from build123d import *

# Parameters (mm, degrees)
SKICA1_W                = 7.9
SKICA1_H                = 3
P_IDAT_VYSUNUT_M1_DEPTH = 2.3
SKICA2_R                = 1
P_IDAT_VYSUNUT_M2_DEPTH = 2.5
ZKOSEN_2_SIZE           = 0.7


with BuildPart() as part:
    # Skica1 → Přidat vysunutím1 (new body)
    with BuildSketch(Plane.XY):
        Rectangle(SKICA1_W, SKICA1_H)
    extrude(amount=P_IDAT_VYSUNUT_M1_DEPTH)

    # Skica2 → Přidat vysunutím2 (add)
    with BuildSketch(Plane.XY.offset(2.3)):
        with Locations((-2.3, 0)):
            Circle(SKICA2_R)
        with Locations((2.3, 0)):
            Circle(SKICA2_R)
    extrude(amount=P_IDAT_VYSUNUT_M2_DEPTH)

    # Zkosení2
    zkosen_2_edges = [part.edges().sort_by_distance(p)[0] for p in [
        (-3.3, 0, 4.8),
        (1.3, 0, 4.8),
    ]]
    chamfer(zkosen_2_edges, length=ZKOSEN_2_SIZE)


solid = part.part
Input: part model. Units: mm. Frame: model coordinates. A direction names the side the tool comes from. Coordinates: 2 decimals unless noted, no trailing zeros. Loops run counter-clockwise (first coordinate to the right, second up) from the corner with the lowest first, then second, coordinate; pieces in that order, holes last. Notation, with made-up numbers: (-20.75, -2.5) -> (-6.75, -2.5) arc R16 cw to (-6.75, 20.5) -> close; hole circle Ø8 at (11.5, 45.5). An arc over 180 degrees is marked (long way). Write each question's results on one line, items separated by ' | '. Start each with the question number.
Q1. Pin query (flat end, axial travel): pin 1 (0.9 mm diameter, centred on x = 0.5, y = 0, fed in from +Z). Return the tip coordinate at first contact, or that it passes through.
Q2. Reachability of faces 1 (the cylindrical face through (-3.3, 0, 3.2)), 2 (the flat face through (3.95, 0, 1)) from +Z, -Z, +X, -X, +Y, -Y: full face, straight path, thin tool, end or side. Return the list, or none.
Q3. Section A-A, the plane y = 0. Return the cut outline in (x, z), plus the area to 3 significant figures.
Q4. Section C-C, the plane x = 2.3. Return the cut outline in (y, z).
Q5. Pull-direction query (X, two-part tool) for faces 3 (the flat face through (-3.95, 0, 1)), 4 (the flat face through (0, 0, 2.3)), 5 (the flat face through (0, -1.5, 1)); classes: released by +X, released by -X, zero draft, split by the parting line, or undercut.
Q6. Section B-B, the plane z = 4.4. Return the cut outline in (x, y).
Q7. Section D-D, the plane z = 3.65. Return the cut outline in (x, y), plus the area to 3 significant figures.
Q8. Ray query, line 1 (Z direction, x = 0, y = -0.15); line 2 (X direction, y = 0.8, z = 3); line 3 (X direction, y = -0.6, z = 3.8). Return the intervals inside material, ascending. Write a range as from..to.
Found:
1) pin 1: z = 2.3
2) face 1: +Z | face 2: +Z, -Z, +X, +Y, -Y
3) outline: (-3.95, 0) -> (3.95, 0) -> (3.95, 2.3) -> (3.3, 2.3) -> (3.3, 4.1) -> (2.6, 4.8) -> (2, 4.8) -> (1.3, 4.1) -> (1.3, 2.3) -> (-1.3, 2.3) -> (-1.3, 4.1) -> (-2, 4.8) -> (-2.6, 4.8) -> (-3.3, 4.1) -> (-3.3, 2.3) -> (-3.95, 2.3) -> close | area: 27.2 mm2
4) outline: (-1.5, 0) -> (1.5, 0) -> (1.5, 2.3) -> (1, 2.3) -> (1, 4.1) -> (0.3, 4.8) -> (-0.3, 4.8) -> (-1, 4.1) -> (-1, 2.3) -> (-1.5, 2.3) -> close
5) face 3: released by -X | face 4: undercut | face 5: zero draft
6) outline: circle Ø1.4 at (-2.3, 0); circle Ø1.4 at (2.3, 0)
7) outline: circle Ø2 at (-2.3, 0); circle Ø2 at (2.3, 0) | area: 6.28 mm2
8) line 1: 0..2.3 | line 2: -2.9..-1.7, 1.7..2.9 | line 3: -3.1..-1.5, 1.5..3.1
